Check sheet for the drawn part. Datum: minimum x, y, z corner. Units: mm. A direction names the side the tool comes from. Coordinates: 2 decimals unless noted, no trailing zeros. Write each loop counter-clockwise with the first axis right and the second up, starting at its lowest first coordinate (ties: lowest second). Pieces come first, ordered by that corner, then holes. Notation, with made-up numbers: (34.5, 83) -> (61.5, 83) arc R22 ccw to (61.5, 103) -> close; hole circle Ø1 at (9.5, 24.5). An arc over 180 degrees is marked (long way). Answer in a Markdown table with one row per item. Add a question column.
1. Mould release check, pull along X, two halves, no side actions. Record for the marked faces 1, 2 and 3: pulls with the +X half, pulls with the -X half, needs draft (parallel to the pull), parting line crosses it, or undercut.
2. Depth check by flat-ended pin: P1, Ø2.5, axis at x = 58.5, y = 20.5, coming from the +Z side; P2, Ø1, axis at y = 36, z = 42, coming from the -X side; P3, Ø3, axis at x = 52.5, z = 21.5, coming from the -Y side. Enter the tip coordinate at first touch or a pass-through.
3. Scan lines: L1, parallel to Z at x = 59, y = 17; L2, parallel to X at y = 6, z = 28; L3, parallel to Z at x = 50, y = 36. Record each from-to range of solid material in increasing order. Write a range as from..to.
4. Cross-section at C-C on x = 10.25. Record the cut outline in (y, z), and give its area (3 significant figures).
5. Cross-section at B-B on z = 45. Record the cut outline in (x, y).
6. Cross-section at D-D on y = 23.5. Record the cut outline in (x, z).
7. Cross-section at A-A on y = 17. Record the cut outline in (x, z).
8. Set-up check for the marked faces 4 and 5: record each of +Z, -Z, +X, -X, +Y, -Y from which the full face is reachable in a straight line by a thin tool's end or side.
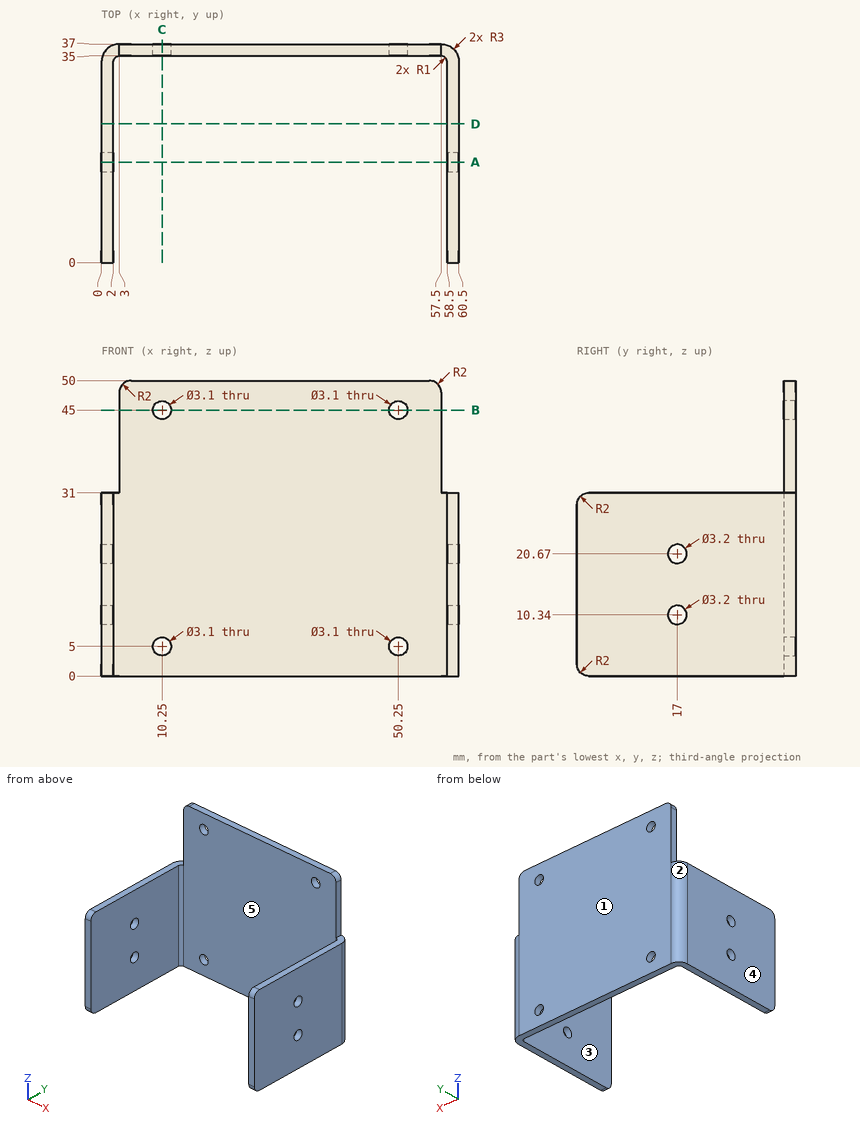
Results found:
| question | item | result |
|---|---|---|
| 1 | face 1 | needs draft |
| 1 | face 2 | pulls with the -X half |
| 1 | face 3 | undercut |
| 2 | P1 | stops at z = 31 |
| 2 | P2 | stops at x = 3 |
| 2 | P3 | stops at y = 35 |
| 3 | L1 | z = 0..8.74, 11.94..19.07, 22.27..31 |
| 3 | L2 | x = 0..2, 58.5..60.5 |
| 3 | L3 | z = 0..3.47, 6.53..43.47, 46.53..50 |
| 4 | outline | (35, 0) -> (37, 0) -> (37, 3.45) -> (35, 3.45) -> close; (35, 6.55) -> (37, 6.55) -> (37, 43.45) -> (35, 43.45) -> close; (35, 46.55) -> (37, 46.55) -> (37, 50) -> (35, 50) -> close |
| 4 | area | 87.6 mm^2 |
| 5 | outline | (3, 35) -> (8.7, 35) -> (8.7, 37) -> (3, 37) -> close; (11.8, 35) -> (48.7, 35) -> (48.7, 37) -> (11.8, 37) -> close; (51.8, 35) -> (57.5, 35) -> (57.5, 37) -> (51.8, 37) -> close |
| 6 | outline | (0, 0) -> (2, 0) -> (2, 31) -> (0, 31) -> close; (58.5, 0) -> (60.5, 0) -> (60.5, 31) -> (58.5, 31) -> close |
| 7 | outline | (0, 0) -> (2, 0) -> (2, 8.74) -> (0, 8.74) -> close; (0, 11.94) -> (2, 11.94) -> (2, 19.07) -> (0, 19.07) -> close; (0, 22.27) -> (2, 22.27) -> (2, 31) -> (0, 31) -> close; (58.5, 0) -> (60.5, 0) -> (60.5, 8.74) -> (58.5, 8.74) -> close; (58.5, 11.94) -> (60.5, 11.94) -> (60.5, 19.07) -> (58.5, 19.07) -> close; (58.5, 22.27) -> (60.5, 22.27) -> (60.5, 31) -> (58.5, 31) -> close |
| 8 | face 4 | +Z, -Z, -X, +Y, -Y |
| 8 | face 5 | +Z, -Z, -Y |
